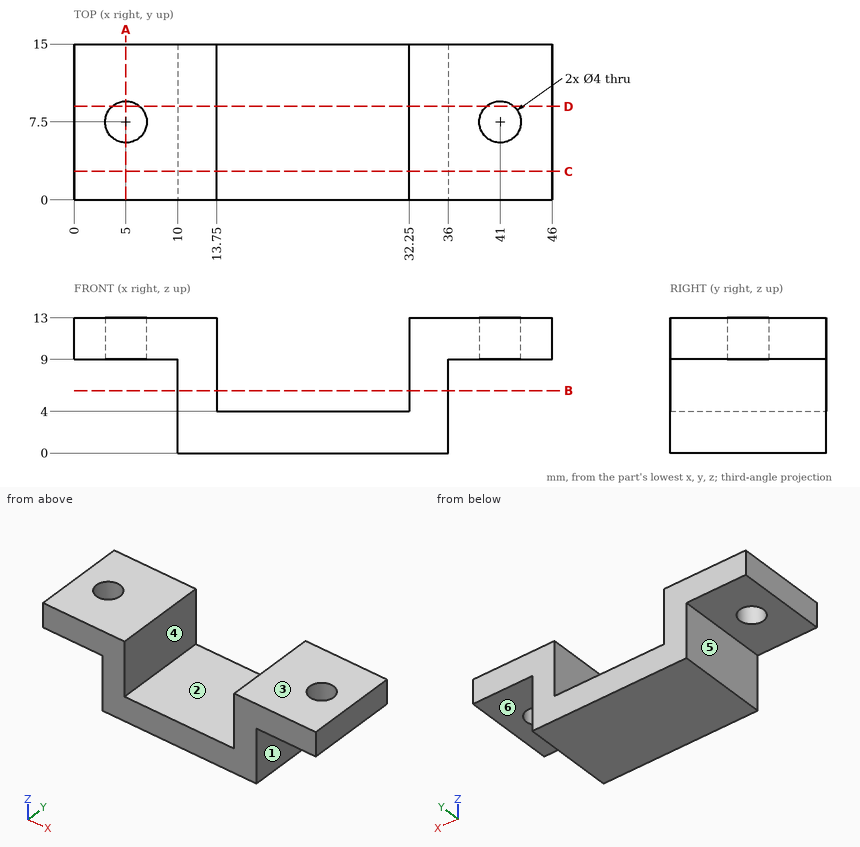
Print and shaded views of the part. All mm, measured from the part's lowest x, y and z. A direction names the side the tool comes from. Give positions to 0.01 mm unless a question says otherwise; leave off trailing zeros. Write each loop counter-clockwise with the first axis right and the second up, starting at its lowest first coordinate (ties: lowest second). Pieces come first, ordered by that corner, then holes. Notation, with made-up numbers: (-23, -5.5) - (23, -5.5) arc R33 cw to (23, 30.5) - close; hole circle Ø5 at (29.5, 15). An arc over 180 degrees is marked (long way). Put each result on its own line as item: value.
(1) Tool access for the marked faces 4, 5 and 6: list every direction of +Z, -Z, +X, -X, +Y, -Y with a clear straight run to the whole face (end or side of a thin tool).
Working result:
face 4: +Z, +Y, -Y
face 5: -Z, -X, +Y, -Y
face 6: -Z, +X, +Y, -Y
(2) Pull direction X, two halves, no side cores. Call the marked faces 1, 2 and 3: released by +X, released by -X, zero draft, split by the parting line, or undercut.
Working result:
face 1: released by +X
face 2: undercut
face 3: zero draft
(3) Saw through at C-C (y = 2.75). List the corners of the cut face in (x, z).
Working result:
outline: (0, 9) - (10, 9) - (10, 0) - (36, 0) - (36, 9) - (46, 9) - (46, 13) - (32.25, 13) - (32.25, 4) - (13.75, 4) - (13.75, 13) - (0, 13) - close
(4) Wall check: L1, parallel to X at y = 7.5, z = 10.4; L2, parallel to X at y = 1.5, z = 4.5; L3, parallel to Y at x = 5, z = 11.65. Give the ranges that are in metal, low to high.
Working result:
L1: 0 to 3, 7 to 13.75, 32.25 to 39, 43 to 46
L2: 10 to 13.75, 32.25 to 36
L3: 0 to 5.5, 9.5 to 15
(5) Drop flat-ended pins along their axis: pin 1 Ø4.5 at (x, y) = (22, 8.5) entering from +Z; pin 2 Ø2.5 at (y, z) = (7.5, 7) entering from +X; pin 3 Ø6.5 at (x, y) = (41, 7.5) entering from -Z. Give the stop position or say it passes through.
Working result:
pin 1: z = 4
pin 2: x = 36
pin 3: z = 9
(6) Saw through at A-A (x = 5). List the corners of the cut face in (y, z), then the cut area to 3 significant figures.
Working result:
outline: (0, 9) - (5.5, 9) - (5.5, 13) - (0, 13) - close; (9.5, 9) - (15, 9) - (15, 13) - (9.5, 13) - close
area: 44.0 mm^2
(7) Saw through at D-D (y = 9). List the corners of the cut face in (x, z), then the cut area to 3 significant figures.
Working result:
outline: (0, 9) - (3.68, 9) - (3.68, 13) - (0, 13) - close; (6.32, 9) - (10, 9) - (10, 0) - (36, 0) - (36, 9) - (39.68, 9) - (39.68, 13) - (32.25, 13) - (32.25, 4) - (13.75, 4) - (13.75, 13) - (6.32, 13) - close; (42.32, 9) - (46, 9) - (46, 13) - (42.32, 13) - close
area: 230 mm^2
(8) Saw through at B-B (z = 6). List the corners of the cut face in (x, y), then the cut area to 4 significant figures.
Working result:
outline: (10, 0) - (13.75, 0) - (13.75, 15) - (10, 15) - close; (32.25, 0) - (36, 0) - (36, 15) - (32.25, 15) - close
area: 112.5 mm^2
